Read the model definition and answer for the solid it produces. Units are mm, in the model's axes. Face numbers are marked on the shaded views. A direction names the side the tool comes from. Round coordinates to 2 decimals unless told otherwise and drop trailing zeros. Loops run counter-clockwise (first coordinate to the right, second up) from the corner with the lowest first, then second, coordinate; pieces in that order, holes last. Notation, with made-up numbers: M 19.5,-21 L 53.5,-21 A11 ccw 53.5,-12 Z; hole C 69,79 d7. An arc over 180 degrees is marked long. Write each question's results on one line, items separated by ' | '.
```python
from build123d import *

# Parameters (mm, degrees)
F2_W     = 15
F2_H     = 10
F3_DEPTH = 30


with BuildPart() as f1:
    # F0 (on Front) → F1 (revolve)
    with BuildSketch(Plane.XZ):
        with BuildLine():
            Line((17.5, 0), (0, 0))
            Line((0, 0), (0, -17.5))
            ThreePointArc((0, -17.5), (12.374369, -12.374369), (17.5, 0))
        make_face()
        Polygon((0, 150), (0, 0), (17.5, 0), (17.5, 10), (16, 10), (16, 80), (17.5, 80), (17.5, 90), (16, 90), (16, 100), (17.5, 100), (17.5, 110), (16, 110), (16, 120), (17.5, 120), (17.5, 130), (16, 130), (16, 140), (17.5, 140), (17.5, 150), align=None)
    revolve(axis=Axis((0, 0, 75), (0, 0, 1)))

    # F2 (on face) → F3 (cut)
    with BuildSketch(Plane.XY.offset(150)):
        Rectangle(F2_W, F2_H)
    extrude(amount=-F3_DEPTH, mode=Mode.SUBTRACT)


solid = f1.part
```
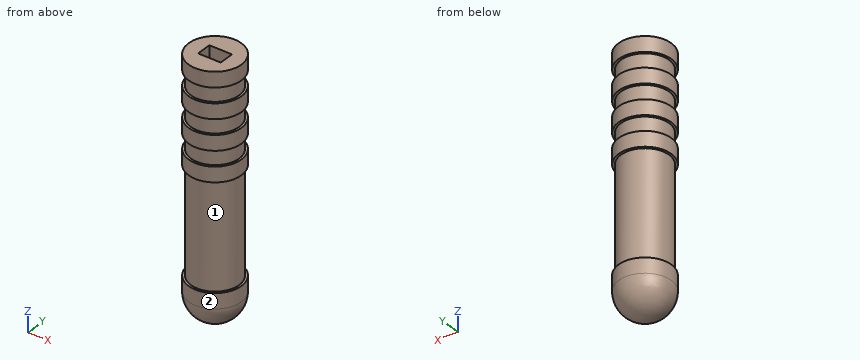
1. Find section A-A, the plane z = 54. Give the vertices of the cut face in (x, y), then the cut area to 3 significant figures.
Completed:
outline: C 0,0 d32 | area: 804 mm2
2. Given P1, Ø5, axis at x = 13, z = 130.5, coming from the -Y side; P2, Ø4, axis at x = -2.5, z = 43.5, coming from the -Y side; P3, Ø4, axis at x = 10, z = 94, coming from the -Y side, each flat-ended and moving along its own axis, determine where each tip first touches the part or whether it passes through.
Completed:
P1: stops at y = -13.96 | P2: stops at y = -15.99 | P3: stops at y = -13.86
3. Which of the six approach directions +Z, -Z, +X, -X, +Y, -Y give full straight-line access (tool end or side, diameter ignored) to the marked faces 1 and 2?
Completed:
face 1: none | face 2: +Z, -Z
4. Find the intervals of material crossed by L1, parallel to X at y = -15, z = -5; L2, parallel to Y at x = 3, z = 136; L3, parallel to Y at x = -5, z = 77.5, in increasing order.
Completed:
L1: x = -7.5 to 7.5 | L2: y = -15.72 to -5, 5 to 15.72 | L3: y = -15.2 to 15.2
